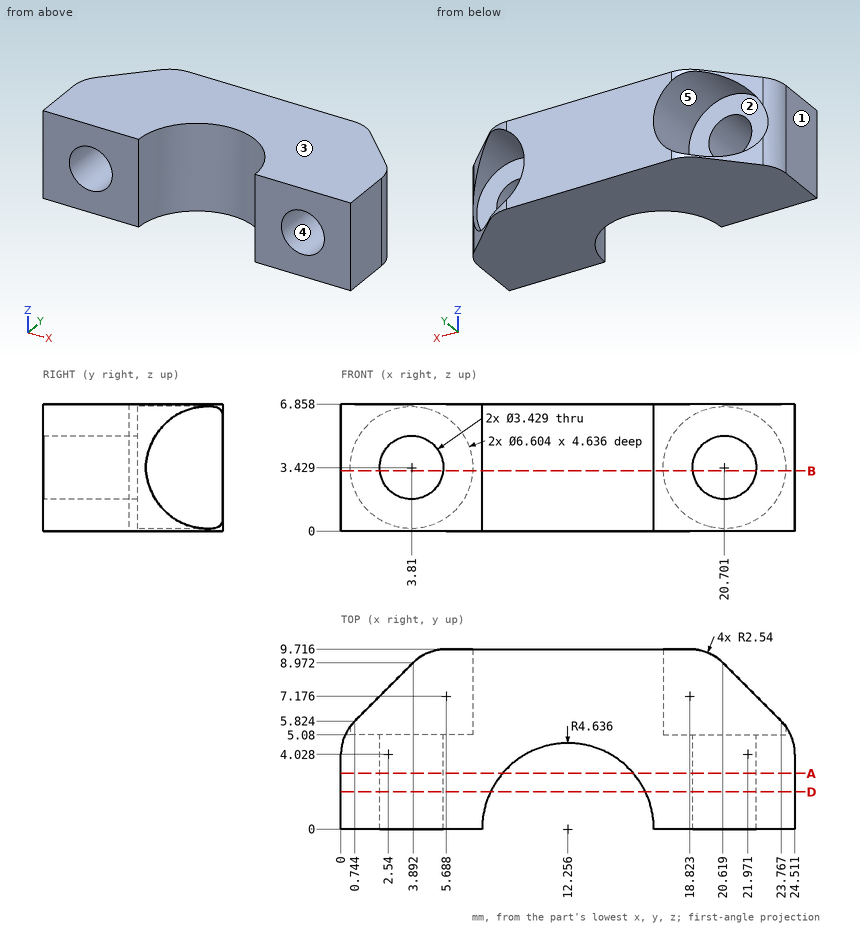
Input: dimensioned drawing with shaded views. Units: mm. Origin: part minimum x, y, z. A direction names the side the tool comes from. Round coordinates to 2 decimals unless told otherwise and drop trailing zeros. Order: outer loops, then holes, each group sorted by start corner. A loop starts at its lowest first (then second) coordinate and runs counter-clockwise, first axis right, second up.
Q1. Section B-B, the plane z = 3.25. Output: boundary loops of the cut face in (x, y) (1 decimal).
Result sheet:
outline: (0, 0) - (2.1, 0) - (2.1, 5.1) - (0.5, 5.1) - (0.5, 5.6) arc R2.5 ccw to (0, 4) - close; (5.5, 0) - (7.6, 0) arc R4.6 cw to (16.9, 0) - (19, 0) - (19, 5.1) - (17.4, 5.1) - (17.4, 9.7) - (7.1, 9.7) - (7.1, 5.1) - (5.5, 5.1) - close; (22.4, 0) - (24.5, 0) - (24.5, 4) arc R2.5 ccw to (24, 5.6) - (24, 5.1) - (22.4, 5.1) - close
Q2. Section A-A, the plane y = 3. Output: boundary loops of the cut face in (x, z) (1 decimal), and give its area (3 significant figures).
Result sheet:
outline: (0, 0) - (8.7, 0) - (8.7, 6.9) - (0, 6.9) - close; (15.8, 0) - (24.5, 0) - (24.5, 6.9) - (15.8, 6.9) - close; hole circle Ø3.4 at (3.8, 3.4); hole circle Ø3.4 at (20.7, 3.4)
area: 101 mm2
Q3. Section D-D, the plane y = 2. Output: boundary loops of the cut face in (x, z) (1 decimal).
Result sheet:
outline: (0, 0) - (8.1, 0) - (8.1, 6.9) - (0, 6.9) - close; (16.4, 0) - (24.5, 0) - (24.5, 6.9) - (16.4, 6.9) - close; hole circle Ø3.4 at (3.8, 3.4); hole circle Ø3.4 at (20.7, 3.4)
Q4. Mould query, pull axis Z, two halves, no side actions, for the marked faces 1, 2 and 3. Classes: released by +Z, released by -Z, zero draft, split by the parting line, or undercut.
Result sheet:
face 1: zero draft
face 2: undercut
face 3: released by +Z
Q5. Pin query (flat end, axial travel): pin 1 (2 mm diameter, centred on x = 20.701, z = 3.429, fed in from +Y); pin 2 (1 mm diameter, centred on x = 3, z = 2, fed in from +Y). Return the tip coordinate at first contact, or that it passes through.
Result sheet:
pin 1: passes through
pin 2: stops at y = 5.08
Q6. Material intervals for probe 1 along Y at (x, z) = (3, 1); probe 2 along X at (y, z) = (1.5, 2.25) (1 decimal); probe 3 along X at (y, z) = (0.75, 1.25), sorted ascending.
Result sheet:
probe 1: y = 0 to 5.08
probe 2: x = 0 to 2.6, 5.1 to 7.9, 16.6 to 19.5, 21.9 to 24.5
probe 3: x = 0 to 7.68, 16.83 to 24.51
Q7. Access query for the marked faces 4 and 5. Directions: +Z, -Z, +X, -X, +Y, -Y. A direction counts if a zero-diameter tool reaches every point of the face in a straight line with its end or side. Return the directions, or none.
Result sheet:
face 4: +Y, -Y
face 5: +Y
